Geometry check sheet. Reference: the model listing, model coordinates, mm. Face numbers are marked on the shaded views. A direction names the side the tool comes from. Coordinates: 2 decimals unless noted, no trailing zeros. Loops run counter-clockwise (first coordinate to the right, second up) from the corner with the lowest first, then second, coordinate; pieces in that order, holes last. Notation, with made-up numbers: (31.5, 14) -> (41.5, 14) arc R21 ccw to (41.5, 30) -> close; hole circle Ø10 at (82, 53.25). An arc over 180 degrees is marked (long way). Answer as a JSON object with one key per item and string values.
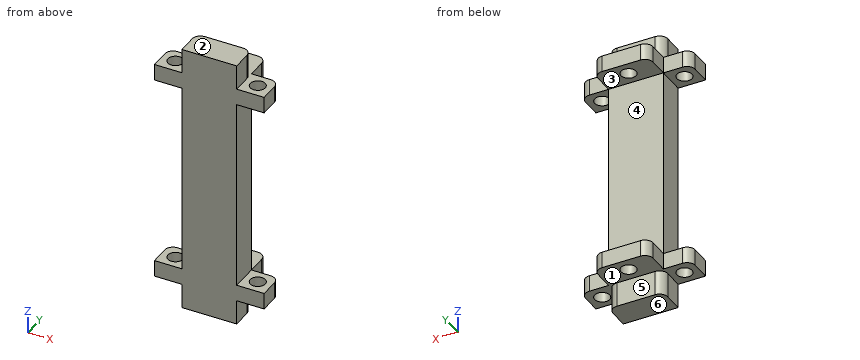
from build123d import *

# Parameters (mm, degrees)
SKETCH_1_W               = 20
SKETCH_1_H               = 10
EXTRUDE_1_DEPTH          = 100
EXTRUDE_START            = -9
SKETCH_2_W               = 10
SKETCH_2_H               = 10
SKETCH_2_W_2             = 20
EXTRUDE_2_DEPTH          = 6
CUT_EXTRUDE_1_DEPTH      = 98.88258272
CUT_EXTRUDE_1_DEPTH_BACK = 98.88258272
SKETCH_3_R               = 2.75
FILLET_1_R               = 3


with BuildPart() as part:
    # 草图1 → 凸台-拉伸1 (new body)
    with BuildSketch(Plane.XY):
        with Locations((10, 5)):
            Rectangle(SKETCH_1_W, SKETCH_1_H)
    extrude(amount=EXTRUDE_1_DEPTH)

    # 草图2 → 凸台-拉伸2 (add)
    with BuildSketch(Plane(origin=(0, 0, 0), x_dir=(-1, 0, 0), z_dir=(0, 0, -1)).offset(EXTRUDE_START)):
        with Locations((-25, 5)):
            Rectangle(SKETCH_2_W, SKETCH_2_H)
        with Locations((-10, 15)):
            Rectangle(SKETCH_2_W_2, SKETCH_2_H)
        with Locations((5, 5)):
            Rectangle(SKETCH_2_W, SKETCH_2_H)
    extrude_2 = extrude(amount=-EXTRUDE_2_DEPTH)

    # 镜向1: 凸台-拉伸2 across plane
    add(extrude_2.mirror(Plane(origin=(0, 0, 50), x_dir=(1, 0, 0), z_dir=(0, 0, -1))))

    # 草图3 → 切除-拉伸1 (cut, two sides: drawn at the far end of the back side and taken through both)
    with BuildSketch(Plane(origin=(0, 0, 9), x_dir=(-1, 0, 0), z_dir=(0, 0, -1)).offset(-CUT_EXTRUDE_1_DEPTH_BACK)):
        with Locations(Location((5, 5, 0), (0, 0, 180))):
            Circle(SKETCH_3_R)
        with Locations(Location((-10, 15, 0), (0, 0, 180))):
            Circle(SKETCH_3_R)
        with Locations(Location((-25, 5, 0), (0, 0, 180))):
            Circle(SKETCH_3_R)
    extrude(amount=CUT_EXTRUDE_1_DEPTH + CUT_EXTRUDE_1_DEPTH_BACK, mode=Mode.SUBTRACT)

    # 圆角1
    # the kernel refuses this fillet: 3 mm, written as the material it takes off along each edge
    with BuildSketch(Plane(origin=(0, 10, -7.5), x_dir=(0, -1, 0), z_dir=(0, 0, 1)), Plane(origin=(0, 10, 91), x_dir=(0, -1, 0), z_dir=(0, 0, 1))) as fillet_1_piece_1:
        with BuildLine():
            CenterArc((FILLET_1_R, FILLET_1_R), FILLET_1_R, 180, 90)
            Line((0, FILLET_1_R), (0, 0))
            Line((0, 0), (FILLET_1_R, 0))
        make_face()
    extrude(amount=16.5, mode=Mode.SUBTRACT)
    with BuildSketch(Plane(origin=(20, 10, -7.5), x_dir=(0, -1, 0), z_dir=(0, 0, 1)), Plane(origin=(20, 10, 91), x_dir=(0, -1, 0), z_dir=(0, 0, 1))) as fillet_1_piece_2:
        with BuildLine():
            CenterArc((FILLET_1_R, -FILLET_1_R), FILLET_1_R, 90, 90)
            Line((0, -FILLET_1_R), (0, 0))
            Line((0, 0), (FILLET_1_R, 0))
        make_face()
    extrude(amount=16.5, mode=Mode.SUBTRACT)
    with BuildSketch(Plane(origin=(20, 20, 1.5), x_dir=(0, -1, 0), z_dir=(0, 0, 1)), Plane(origin=(30, 10, 1.5), x_dir=(0, -1, 0), z_dir=(0, 0, 1)), Plane(origin=(0, 20, 98.5), x_dir=(0, -1, 0), z_dir=(0, 0, -1)), Plane(origin=(-10, 10, 98.5), x_dir=(0, -1, 0), z_dir=(0, 0, -1))) as fillet_1_piece_3:
        with BuildLine():
            CenterArc((FILLET_1_R, -FILLET_1_R), FILLET_1_R, 90, 90)
            Line((0, -FILLET_1_R), (0, 0))
            Line((0, 0), (FILLET_1_R, 0))
        make_face()
    extrude(amount=21, mode=Mode.SUBTRACT)
    with BuildSketch(Plane(origin=(0, 20, 1.5), x_dir=(0, -1, 0), z_dir=(0, 0, 1)), Plane(origin=(-10, 10, 1.5), x_dir=(0, -1, 0), z_dir=(0, 0, 1)), Plane(origin=(30, 10, 98.5), x_dir=(0, -1, 0), z_dir=(0, 0, -1)), Plane(origin=(20, 20, 98.5), x_dir=(0, -1, 0), z_dir=(0, 0, -1))) as fillet_1_piece_4:
        with BuildLine():
            CenterArc((FILLET_1_R, FILLET_1_R), FILLET_1_R, 180, 90)
            Line((0, FILLET_1_R), (0, 0))
            Line((0, 0), (FILLET_1_R, 0))
        make_face()
    extrude(amount=21, mode=Mode.SUBTRACT)


solid = part.part
1. Section check D-D, the plane z = 47. Record the boundary of the cut face in (x, y).
Evaluation:
{"outline": "(0, 0) -> (20, 0) -> (20, 10) -> (0, 10) -> close"}
2. Depth check by flat-ended pin: P1, Ø5, axis at x = 10, y = 13.5, coming from the +Z side; P2, Ø3.5, axis at y = 3.5, z = 93.5, coming from the +X side; P3, Ø2, axis at y = 6, z = 17, coming from the -X side. Enter the tip coordinate at first touch or a pass-through.
Evaluation:
{"P1": "stops at z = 91", "P2": "stops at x = 20", "P3": "stops at x = 0"}
3. Section check A-A, the plane x = 10. Record the boundary of the cut face in (y, z), then the cut area to 3 significant figures.
Evaluation:
{"outline": "(0, 0) -> (10, 0) -> (10, 9) -> (12.25, 9) -> (12.25, 15) -> (10, 15) -> (10, 85) -> (12.25, 85) -> (12.25, 91) -> (10, 91) -> (10, 100) -> (0, 100) -> close; (17.75, 9) -> (20, 9) -> (20, 15) -> (17.75, 15) -> close; (17.75, 85) -> (20, 85) -> (20, 91) -> (17.75, 91) -> close", "area": "1,050 mm^2"}
4. Section check B-B, the plane x = 25. Record the boundary of the cut face in (y, z), then the cut area to 3 significant figures.
Evaluation:
{"outline": "(0, 9) -> (2.25, 9) -> (2.25, 15) -> (0, 15) -> close; (0, 85) -> (2.25, 85) -> (2.25, 91) -> (0, 91) -> close; (7.75, 9) -> (10, 9) -> (10, 15) -> (7.75, 15) -> close; (7.75, 85) -> (10, 85) -> (10, 91) -> (7.75, 91) -> close", "area": "54.0 mm^2"}
5. Thickness scan on probe 1 along Y at (x, z) = (10, 12.35); probe 2 along Z at (x, y) = (19.5, 15.25); probe 3 along Y at (x, z) = (7.5, 26). Record the ranges inside material, lowest first. Write a range as from..to.
Evaluation:
{"probe 1": "y = 0..12.25, 17.75..20", "probe 2": "z = 9..15, 85..91", "probe 3": "y = 0..10"}
6. Mould release check, pull along Z, two halves, no side actions. Record for the marked faces 4, 5 and 6: released by +Z, released by -Z, zero draft, split by the parting line, or undercut.
Evaluation:
{"face 4": "undercut", "face 5": "zero draft", "face 6": "released by -Z"}
7. Tool access check on the marked faces 1, 2 and 3. Record the directions out of +Z, -Z, +X, -X, +Y, -Y that give a thin tool (end or side, any length) a straight path to the whole face; none if there is none.
Evaluation:
{"face 1": "-Z, +Y", "face 2": "+Z, +X, -X, +Y, -Y", "face 3": "+X, -X, +Y"}
8. Section check C-C, the plane y = 13.25. Record the boundary of the cut face in (x, z).
Evaluation:
{"outline": "(0, 9) -> (7.88, 9) -> (7.88, 15) -> (0, 15) -> close; (0, 85) -> (7.88, 85) -> (7.88, 91) -> (0, 91) -> close; (12.12, 9) -> (20, 9) -> (20, 15) -> (12.12, 15) -> close; (12.12, 85) -> (20, 85) -> (20, 91) -> (12.12, 91) -> close"}
